from build123d import *

# Parameters (mm, degrees)
SKETCH1_W           = 15
SKETCH1_H           = 18.6
SKETCH1_R           = 1.25
BOSS_EXTRUDE1_DEPTH = 1.4
SKETCH3_RX          = 1.238007016
SKETCH3_RY          = 0.65851437
BOSS_EXTRUDE2_DEPTH = 11.6
SKETCH4_W           = 0.456640639
SKETCH4_H           = 9.610469394
SKETCH4_W_2         = 0.530038758
SKETCH4_W_3         = 2.48112331
SKETCH4_W_4         = 2.853524762
CUT_EXTRUDE1_DEPTH  = 18.6
CUT_EXTRUDE2_REACH  = 29.202
SKETCH5_W           = 9.610469394
SKETCH5_H           = 4.489024126
SKETCH5_H_2         = 2.452224348


with BuildPart() as part:
    # Sketch1 → Boss-Extrude1 (new body)
    with BuildSketch(Plane.XY):
        with Locations((7.5, 9.3)):
            Rectangle(SKETCH1_W, SKETCH1_H)
        with Locations((2.25, 16.85)):
            Circle(SKETCH1_R, mode=Mode.SUBTRACT)
        with Locations(Location((12.75, 16.85, 0), (0, 0, 180))):
            Circle(SKETCH1_R, mode=Mode.SUBTRACT)
    extrude(amount=BOSS_EXTRUDE1_DEPTH)

    # Sketch3 → Boss-Extrude2 (add)
    with BuildSketch(Plane.XY.offset(1.4)):
        with Locations(Location((7.5, 9.3), (0, 0, 180))):
            Ellipse(SKETCH3_RX, SKETCH3_RY)
    extrude(amount=BOSS_EXTRUDE2_DEPTH)

    # Sketch4 → Cut-Extrude1 (cut)
    with BuildSketch(Plane.XZ):
        with Locations((7.087370884, 6.205234697)):
            Rectangle(SKETCH4_W, SKETCH4_H)
        with Locations((8.008203946, 6.205234697)):
            Rectangle(SKETCH4_W_2, SKETCH4_H)
        with Locations((5.200227297, 6.205234697)):
            Rectangle(SKETCH4_W_3, SKETCH4_H)
        with Locations((9.992974241, 6.205234697)):
            Rectangle(SKETCH4_W_4, SKETCH4_H)
    extrude(amount=-CUT_EXTRUDE1_DEPTH, mode=Mode.SUBTRACT)

    # Cut-Extrude2: up to this face of the body (flat: up to its plane)
    cut_extrude2_end = Plane(part.part.faces().sort_by_distance((15, 9.3, 0.7))[0])
    # Sketch5 → Cut-Extrude2 (cut, up to the picked face)
    with BuildSketch(Plane.ZY, mode=Mode.PRIVATE) as cut_extrude2_sk1:
        with Locations((6.205234697, 11.811177541)):
            Rectangle(SKETCH5_W, SKETCH5_H)
    cut_extrude2_tool1 = split(extrude(cut_extrude2_sk1.sketch, amount=-CUT_EXTRUDE2_REACH, mode=Mode.PRIVATE), bisect_by=cut_extrude2_end, keep=Keep.BOTH, mode=Mode.PRIVATE)
    # Sketch5 → Cut-Extrude2 (cut, up to the picked face)
    with BuildSketch(Plane.ZY, mode=Mode.PRIVATE) as cut_extrude2_sk2:
        with Locations((6.205234697, 7.887207935)):
            Rectangle(SKETCH5_W, SKETCH5_H_2)
    cut_extrude2_tool2 = split(extrude(cut_extrude2_sk2.sketch, amount=-CUT_EXTRUDE2_REACH, mode=Mode.PRIVATE), bisect_by=cut_extrude2_end, keep=Keep.BOTH, mode=Mode.PRIVATE)
    add(cut_extrude2_tool1.solids().sort_by(Axis((0, 11.811178, 6.205235), (1, 0, 0)))[0], mode=Mode.SUBTRACT)
    add(cut_extrude2_tool2.solids().sort_by(Axis((0, 7.887208, 6.205235), (1, 0, 0)))[0], mode=Mode.SUBTRACT)


solid = part.part
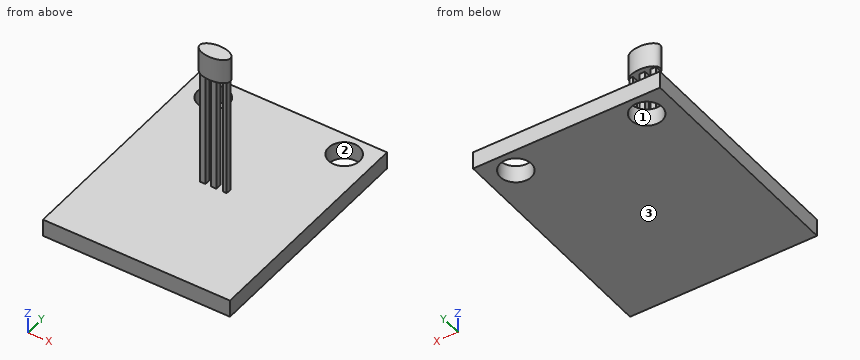
Here's how the part is built. I have some questions about the finished solid (model axes, mm). Face numbers are marked on the shaded views. Coordinates: 2 decimals unless noted, no trailing zeros. Order: outer loops, then holes, each group sorted by start corner. A loop starts at its lowest first (then second) coordinate and runs counter-clockwise, first axis right, second up.
Item 1: If we section it at A-A on x = 12.75: List the corners of the cut face in (y, z) for me.
Result sheet:
outline: (0, 0) - (15.6, 0) - (15.6, 1.4) - (0, 1.4) - close; (18.1, 0) - (18.6, 0) - (18.6, 1.4) - (18.1, 1.4) - close
Item 2: For P1, Ø0.5, axis at x = 7.5, z = 5, coming from the -Y side; P2, Ø0.5, axis at y = 9.5, z = 6.5, coming from the +X side; P3, Ø3, axis at x = 12.75, y = 16.85, coming from the +Z side, each with a flat end and sliding along its axis, tell me the tip position at first contact or that it passes through.
Result sheet:
P1: stops at y = 9.11
P2: stops at x = 8.57
P3: stops at z = 1.4
Item 3: If we mould it in two halves opening along X, with no side actions, what happens to the marked faces 1, 2 and 3? For each: +X half, -X half, draft (parallel to the pull), parting line (faces both ways), or undercut.
Result sheet:
face 1: undercut
face 2: undercut
face 3: draft
Item 4: If we section it at B-B on y = 16.5: List the corners of the cut face in (x, z) for me.
Result sheet:
outline: (0, 0) - (1.05, 0) - (1.05, 1.4) - (0, 1.4) - close; (3.45, 0) - (11.55, 0) - (11.55, 1.4) - (3.45, 1.4) - close; (13.95, 0) - (15, 0) - (15, 1.4) - (13.95, 1.4) - close
Item 5: I need wall thicknesses on line 1 (Y direction, x = 2.25, z = 1.1); line 2 (Z direction, x = 4.5, y = 8.75); line 3 (Y direction, x = 7.5, z = 2.25). Which ranges of each line are inside material? Lowest first, please.
Result sheet:
line 1: y = 0 to 15.6, 18.1 to 18.6
line 2: z = 0 to 1.4
line 3: y = 9.11 to 9.57
Item 6: If we section it at C-C on z = 3: List the corners of the cut face in (x, y) for me.
Result sheet:
outline: (6.44, 9.11) - (6.86, 9.11) - (6.86, 9.57) - (6.44, 9.57) - close; (7.32, 9.11) - (7.74, 9.11) - (7.74, 9.57) - (7.32, 9.57) - close; (8.27, 9.11) - (8.57, 9.11) - (8.57, 9.57) - (8.27, 9.57) - close
Item 7: If we section it at D-D on x = 9.25: List the corners of the cut face in (y, z) for me.
Result sheet:
outline: (0, 0) - (18.6, 0) - (18.6, 1.4) - (0, 1.4) - close
